Part model, mm, in its own coordinate system. Coordinates: 2 decimals unless noted, no trailing zeros. Write each loop counter-clockwise with the first axis right and the second up, starting at its lowest first coordinate (ties: lowest second). Pieces come first, ordered by that corner, then holes. Notation, with made-up numbers: (84.5, 8) - (115.5, 8) arc R3 cw to (115.5, 13) - close; hole circle Ø6 at (2, -5). An arc over 180 degrees is marked (long way). Use a Markdown table: item, result.
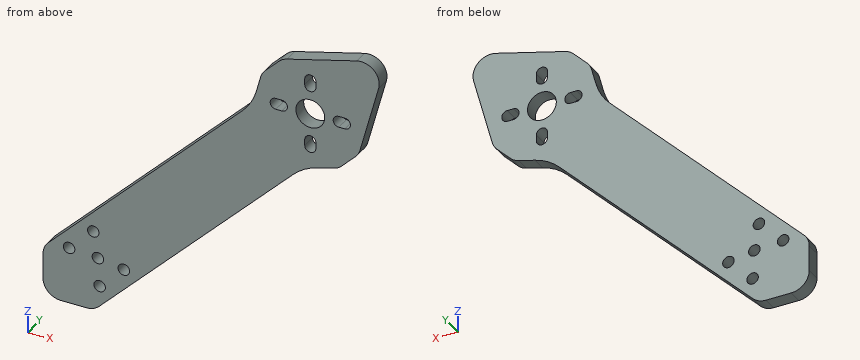
```python
from build123d import *

# Parameters (mm, degrees)
F0_R     = 1.6
F0_R_2   = 4
F1_DEPTH = 4


with BuildPart() as f1:
    # F0 (on Front) → F1 (new body)
    with BuildSketch(Plane.XZ):
        with BuildLine():
            Line((55.367359, 69.509495), (1.464466, 15.606602))
            ThreePointArc((1.464466, 15.606602), (0.380602, 13.984485), (0, 12.071068))
            Line((0, 12.071068), (0, 5))
            ThreePointArc((0, 5), (1.464466, 1.464466), (5, 0))
            Line((5, 0), (12.071068, 0))
            ThreePointArc((12.071068, 0), (13.984485, 0.380602), (15.606602, 1.464466))
            Line((15.606602, 1.464466), (69.509495, 55.367359))
            ThreePointArc((69.509495, 55.367359), (72.616096, 57.751138), (76.233811, 59.249645))
            Line((76.233811, 59.249645), (80.716688, 60.450828))
            ThreePointArc((80.716688, 60.450828), (81.922593, 60.95033), (82.958127, 61.744923))
            Line((82.958127, 61.744923), (86.747501, 65.534297))
            ThreePointArc((86.747501, 65.534297), (87.542094, 66.569831), (88.041596, 67.775736))
            Line((88.041596, 67.775736), (93.217977, 87.094252))
            ThreePointArc((93.217977, 87.094252), (91.923882, 91.923882), (87.094252, 93.217977))
            Line((87.094252, 93.217977), (67.775736, 88.041596))
            ThreePointArc((67.775736, 88.041596), (66.569831, 87.542094), (65.534297, 86.747501))
            Line((65.534297, 86.747501), (61.744923, 82.958127))
            ThreePointArc((61.744923, 82.958127), (60.95033, 81.922593), (60.450828, 80.716688))
            Line((60.450828, 80.716688), (59.249645, 76.233811))
            ThreePointArc((59.249645, 76.233811), (57.751138, 72.616096), (55.367359, 69.509495))
        make_face()
        with Locations((15.734, 7.322)):
            Circle(F0_R, mode=Mode.SUBTRACT)
        with Locations((7.249, 15.807)):
            Circle(F0_R, mode=Mode.SUBTRACT)
        with Locations((15.25, 15.25)):
            Circle(F0_R, mode=Mode.SUBTRACT)
        with Locations((22.452, 14.039)):
            Circle(F0_R, mode=Mode.SUBTRACT)
        with Locations((13.966, 22.524)):
            Circle(F0_R, mode=Mode.SUBTRACT)
        with BuildLine():
            ThreePointArc((75.796212, 64.646212), (74.246212, 63.096212), (72.696212, 64.646212))
            Line((72.696212, 64.646212), (72.696212, 66.346212))
            ThreePointArc((72.696212, 66.346212), (74.246212, 67.896212), (75.796212, 66.346212))
            Line((75.796212, 66.346212), (75.796212, 64.646212))
        make_face(mode=Mode.SUBTRACT)
        with BuildLine():
            ThreePointArc((64.646212, 72.696212), (63.096212, 74.246212), (64.646212, 75.796212))
            Line((64.646212, 75.796212), (66.346212, 75.796212))
            ThreePointArc((66.346212, 75.796212), (67.896212, 74.246212), (66.346212, 72.696212))
            Line((66.346212, 72.696212), (64.646212, 72.696212))
        make_face(mode=Mode.SUBTRACT)
        with Locations((74.246212, 74.246212)):
            Circle(F0_R_2, mode=Mode.SUBTRACT)
        with BuildLine():
            ThreePointArc((83.846212, 75.796212), (85.396212, 74.246212), (83.846212, 72.696212))
            Line((83.846212, 72.696212), (82.146212, 72.696212))
            ThreePointArc((82.146212, 72.696212), (80.596212, 74.246212), (82.146212, 75.796212))
            Line((82.146212, 75.796212), (83.846212, 75.796212))
        make_face(mode=Mode.SUBTRACT)
        with BuildLine():
            ThreePointArc((72.696212, 83.846212), (74.246212, 85.396212), (75.796212, 83.846212))
            Line((75.796212, 83.846212), (75.796212, 82.146212))
            ThreePointArc((75.796212, 82.146212), (74.246212, 80.596212), (72.696212, 82.146212))
            Line((72.696212, 82.146212), (72.696212, 83.846212))
        make_face(mode=Mode.SUBTRACT)
    extrude(amount=F1_DEPTH)


solid = f1.part
```
Item 1: Drop flat-ended pins along their axis: P1, Ø1.4, axis at x = 65.5, y = -2.5, coming from the -Z side; P2, Ø0.5, axis at y = -2, z = 65, coming from the -X side; P3, Ø0.5, axis at x = 83.5, y = -2, coming from the -Z side; P4, Ø2.5, axis at x = 22.452, z = 14.039, coming from the -Y side. Give the stop position or say it passes through.
From the geometry:
| item | result |
|---|---|
| P1 | z = 50.66 |
| P2 | x = 50.61 |
| P3 | z = 62.04 |
| P4 | through |
Item 2: Band-saw the part on C-C, the plane x = 41. Give the cut face in (y, z), then the cut area to 3 significant figures.
From the geometry:
| item | result |
|---|---|
| outline | (-4, 26.86) - (0, 26.86) - (0, 55.14) - (-4, 55.14) - close |
| area | 113 mm^2 |
Item 3: Band-saw the part on B-B, the plane z = 26. Give the cut face in (x, y).
From the geometry:
| item | result |
|---|---|
| outline | (11.86, -4) - (40.14, -4) - (40.14, 0) - (11.86, 0) - close |
Item 4: Drill centre lines: probe 1 along X at (y, z) = (-2.35, 73); probe 2 along Z at (x, y) = (23.5, -0.7); probe 3 along X at (y, z) = (-0.85, 22). Where is each one in solid material? Low to high.
From the geometry:
| item | result |
|---|---|
| probe 1 | 57.97 to 63.72, 67.27 to 70.45, 78.05 to 81.22, 84.77 to 89.44 |
| probe 2 | 9.36 to 12.83, 15.25 to 37.64 |
| probe 3 | 7.86 to 12.45, 15.48 to 36.14 |
Item 5: Band-saw the part on A-A, the plane y = -1.5. Count the separate pieces of the cut face and the enclosed holes in it, then the cut area to 3 significant figures.
From the geometry:
| item | result |
|---|---|
| separate pieces | 1 |
| enclosed holes | 10 |
| area | 2,430 mm^2 |
